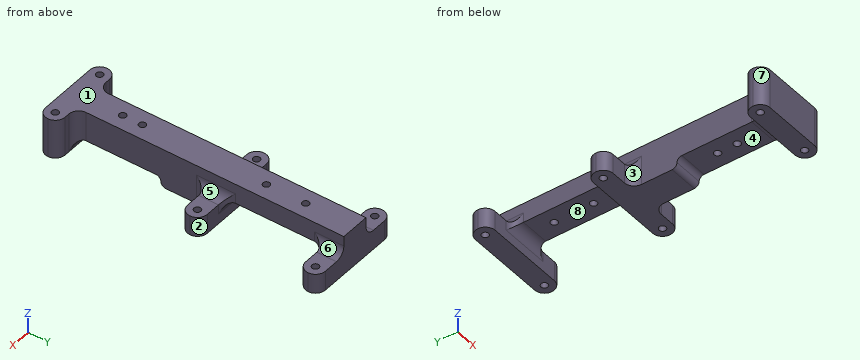
```python
from build123d import *

# Parameters (mm, degrees)
SKETCH1_W                = 50
SKETCH1_H                = 10
BOSS_EXTRUDE1_DEPTH      = 10
BOSS_EXTRUDE1_2_DEPTH    = 10
SKETCH2_W                = 15
SKETCH2_H                = 70
BOSS_EXTRUDE2_DEPTH      = 10
CUT_EXTRUDE1_REACH       = 49.434
SKETCH3_R                = 1.75
CUT_EXTRUDE2_REACH       = 46.159
SKETCH4_R                = 1.75
FILLET2_R                = 5
FILLET4_R                = 5
FILLET5_R                = 5
FILLET6_R                = 5
SKETCH5_W                = 15
SKETCH5_H                = 20
BOSS_EXTRUDE3_DEPTH      = 66
BOSS_EXTRUDE4_DEPTH      = 20
BOSS_EXTRUDE4_DEPTH_BACK = 20
SKETCH6_W                = 20
SKETCH6_H                = 10
CUT_EXTRUDE3_REACH       = 117.525
SKETCH7_R                = 1.75
FILLET7_R                = 5
FILLET9_R                = 5
FILLET10_R               = 5
SKETCH8_R                = 1.75
CUT_EXTRUDE4_DEPTH       = 116.524889093
SKETCH11_W               = 15
SKETCH11_H               = 43
CUT_EXTRUDE5_DEPTH       = 5
FILLET11_R               = 5
FILLET13_R               = 2.5


# Some blends are built 0.0001 mm under size
with BuildPart() as part:
    # Sketch1 → Boss-Extrude1 (new body)
    with BuildSketch(Plane.XY):
        with Locations((0, 30)):
            Rectangle(SKETCH1_W, SKETCH1_H)
    extrude(amount=BOSS_EXTRUDE1_DEPTH)



with BuildPart() as body_2:
    # Sketch1 → Boss-Extrude1 2 (new body)
    with BuildSketch(Plane.XY):
        with Locations((0, -30)):
            Rectangle(SKETCH1_W, SKETCH1_H)
    extrude(amount=BOSS_EXTRUDE1_2_DEPTH)


with BuildPart() as part_1:
    add(part.part)

    add(body_2.part)  # Boss-Extrude2 merges body 2
    # Sketch2 → Boss-Extrude2 (add)
    with BuildSketch(Plane.XY.offset(10)):
        Rectangle(SKETCH2_W, SKETCH2_H)
    extrude(amount=BOSS_EXTRUDE2_DEPTH)

    # Sketch3 → Cut-Extrude1 (cut, up to next)
    with BuildSketch(Plane.XY.offset(20), mode=Mode.PRIVATE) as cut_extrude1_sk1:
        with Locations((0, 10)):
            Circle(SKETCH3_R)
    cut_extrude1_tool1 = extrude(cut_extrude1_sk1.sketch, amount=-CUT_EXTRUDE1_REACH, mode=Mode.PRIVATE) & part_1.part
    # Sketch3 → Cut-Extrude1 (cut, up to next)
    with BuildSketch(Plane.XY.offset(20), mode=Mode.PRIVATE) as cut_extrude1_sk2:
        with Locations((0, -10)):
            Circle(SKETCH3_R)
    cut_extrude1_tool2 = extrude(cut_extrude1_sk2.sketch, amount=-CUT_EXTRUDE1_REACH, mode=Mode.PRIVATE) & part_1.part
    add(cut_extrude1_tool1.solids().sort_by_distance((0, 10, 20))[0], mode=Mode.SUBTRACT)
    add(cut_extrude1_tool2.solids().sort_by_distance((0, -10, 20))[0], mode=Mode.SUBTRACT)

    # Sketch4 → Cut-Extrude2 (cut, up to next)
    with BuildSketch(Plane.XY.offset(10), mode=Mode.PRIVATE) as cut_extrude2_sk1:
        with Locations((-20, 30)):
            Circle(SKETCH4_R)
    cut_extrude2_tool1 = extrude(cut_extrude2_sk1.sketch, amount=-CUT_EXTRUDE2_REACH, mode=Mode.PRIVATE) & part_1.part
    # Sketch4 → Cut-Extrude2 (cut, up to next)
    with BuildSketch(Plane.XY.offset(10), mode=Mode.PRIVATE) as cut_extrude2_sk2:
        with Locations((-20, -30)):
            Circle(SKETCH4_R)
    cut_extrude2_tool2 = extrude(cut_extrude2_sk2.sketch, amount=-CUT_EXTRUDE2_REACH, mode=Mode.PRIVATE) & part_1.part
    # Sketch4 → Cut-Extrude2 (cut, up to next)
    with BuildSketch(Plane.XY.offset(10), mode=Mode.PRIVATE) as cut_extrude2_sk3:
        with Locations((20, 30)):
            Circle(SKETCH4_R)
    cut_extrude2_tool3 = extrude(cut_extrude2_sk3.sketch, amount=-CUT_EXTRUDE2_REACH, mode=Mode.PRIVATE) & part_1.part
    # Sketch4 → Cut-Extrude2 (cut, up to next)
    with BuildSketch(Plane.XY.offset(10), mode=Mode.PRIVATE) as cut_extrude2_sk4:
        with Locations((20, -30)):
            Circle(SKETCH4_R)
    cut_extrude2_tool4 = extrude(cut_extrude2_sk4.sketch, amount=-CUT_EXTRUDE2_REACH, mode=Mode.PRIVATE) & part_1.part
    add(cut_extrude2_tool1.solids().sort_by_distance((-20, 30, 10))[0], mode=Mode.SUBTRACT)
    add(cut_extrude2_tool2.solids().sort_by_distance((-20, -30, 10))[0], mode=Mode.SUBTRACT)
    add(cut_extrude2_tool3.solids().sort_by_distance((20, 30, 10))[0], mode=Mode.SUBTRACT)
    add(cut_extrude2_tool4.solids().sort_by_distance((20, -30, 10))[0], mode=Mode.SUBTRACT)

    # Fillet2
    fillet2_edges = [part_1.edges().sort_by_distance(p)[0] for p in [
        (25, -35, 5),
        (25, -25, 5),
        (25, 35, 5),
        (25, 25, 5),
        (-25, 35, 5),
        (-25, 25, 5),
        (-25, -25, 5),
        (-25, -35, 5),
    ]]
    fillet(fillet2_edges, radius=FILLET2_R - 0.0001)  # a hair under: the kernel refuses the full size

    # Fillet4
    # the kernel refuses this fillet: 5 mm, written as the material it adds along each edge
    with BuildSketch(Plane(origin=(7.5, 25, 10), x_dir=(0, 0, -1), z_dir=(-1, 0, 0))) as fillet4_piece_1:
        with BuildLine():
            CenterArc((FILLET4_R, FILLET4_R), FILLET4_R, 180, 90)
            Line((0, FILLET4_R), (0, 0))
            Line((0, 0), (FILLET4_R, 0))
        make_face()
    extrude(amount=15)
    with BuildSketch(Plane(origin=(-7.5, -25, 10), x_dir=(0, 1, 0), z_dir=(1, 0, 0))) as fillet4_piece_2:
        with BuildLine():
            CenterArc((FILLET4_R, -FILLET4_R), FILLET4_R, 90, 90)
            Line((0, -FILLET4_R), (0, 0))
            Line((0, 0), (FILLET4_R, 0))
        make_face()
    extrude(amount=15)

    # Fillet5
    fillet5_edges = [part_1.edges().sort_by_distance(p)[0] for p in [
        (7.5, -25, 7.5),
        (7.5, 25, 7.5),
    ]]
    fillet(fillet5_edges, radius=FILLET5_R - 0.0001)  # a hair under: the kernel refuses the full size

    # Fillet6
    fillet6_edges = [part_1.edges().sort_by_distance(p)[0] for p in [
        (-7.5, -25, 7.5),
        (-7.5, 25, 7.5),
    ]]
    fillet(fillet6_edges, radius=FILLET6_R - 0.0001)  # a hair under: the kernel refuses the full size

    # Sketch5 → Boss-Extrude3 (add)
    with BuildSketch(Plane.XZ.offset(35)):
        with Locations((0, 10)):
            Rectangle(SKETCH5_W, SKETCH5_H)
    extrude(amount=BOSS_EXTRUDE3_DEPTH)

    # Sketch6 → Boss-Extrude4 (add, two sides: drawn at the far end of the back side and taken through both)
    with BuildSketch(Plane(origin=(0, 0, 0), x_dir=(0, 0, -1), z_dir=(1, 0, 0)).offset(-BOSS_EXTRUDE4_DEPTH_BACK)):
        with Locations((-10, -106)):
            Rectangle(SKETCH6_W, SKETCH6_H)
    extrude(amount=BOSS_EXTRUDE4_DEPTH + BOSS_EXTRUDE4_DEPTH_BACK)

    # Sketch7 → Cut-Extrude3 (cut, up to next)
    with BuildSketch(Plane.XY.offset(20), mode=Mode.PRIVATE) as cut_extrude3_sk1:
        with Locations((-15, -106)):
            Circle(SKETCH7_R)
    cut_extrude3_tool1 = extrude(cut_extrude3_sk1.sketch, amount=-CUT_EXTRUDE3_REACH, mode=Mode.PRIVATE) & part_1.part
    # Sketch7 → Cut-Extrude3 (cut, up to next)
    with BuildSketch(Plane.XY.offset(20), mode=Mode.PRIVATE) as cut_extrude3_sk2:
        with Locations((15, -106)):
            Circle(SKETCH7_R)
    cut_extrude3_tool2 = extrude(cut_extrude3_sk2.sketch, amount=-CUT_EXTRUDE3_REACH, mode=Mode.PRIVATE) & part_1.part
    add(cut_extrude3_tool1.solids().sort_by_distance((-15, -106, 20))[0], mode=Mode.SUBTRACT)
    add(cut_extrude3_tool2.solids().sort_by_distance((15, -106, 20))[0], mode=Mode.SUBTRACT)

    # Fillet7
    fillet7_edges = [part_1.edges().sort_by_distance(p)[0] for p in [
        (20, -111, 10),
        (20, -101, 10),
        (-20, -111, 10),
        (-20, -101, 10),
    ]]
    fillet(fillet7_edges, radius=FILLET7_R - 0.0001)  # a hair under: the kernel refuses the full size

    # Fillet9
    fillet9_edges = [part_1.edges().sort_by_distance(p)[0] for p in [
        (-7.5, -35, 5),
        (7.5, -35, 5),
    ]]
    fillet(fillet9_edges, radius=FILLET9_R)

    # Fillet10
    fillet10_edges = [part_1.edges().sort_by_distance(p)[0] for p in [
        (7.5, -30.00005, 10),
        (7.5, 27.50005, 10),
        (-7.5, -30.00005, 10),
        (-7.5, 27.50005, 10),
    ]]
    fillet(fillet10_edges, radius=FILLET10_R)

    # Sketch8 → Cut-Extrude4 (cut, through all)
    with BuildSketch(Plane.XY.offset(20)):
        with Locations((0, -73)):
            Circle(SKETCH8_R)
        with Locations((0, -83)):
            Circle(SKETCH8_R)
    extrude(amount=-CUT_EXTRUDE4_DEPTH, mode=Mode.SUBTRACT)

    # Sketch11 → Cut-Extrude5 (cut)
    with BuildSketch(Plane(origin=(0, 0, 0), x_dir=(-1, 0, 0), z_dir=(0, 0, -1))):
        with Locations((0, -79.5)):
            Rectangle(SKETCH11_W, SKETCH11_H)
    extrude(amount=-CUT_EXTRUDE5_DEPTH, mode=Mode.SUBTRACT)

    # Fillet11
    fillet11_edges = [part_1.edges().sort_by_distance(p)[0] for p in [
        (-7.5, -101, 12.5),
        (7.5, -101, 12.5),
        (0, -101, 5),
    ]]
    fillet(fillet11_edges, radius=FILLET11_R - 0.0001)  # a hair under: the kernel refuses the full size

    # Fillet13
    fillet13_edges = [part_1.edges().sort_by_distance(p)[0] for p in [
        (0, -58, 5),
    ]]
    fillet(fillet13_edges, radius=FILLET13_R)
    fillet13_2_edges = [part_1.edges().sort_by_distance(p)[0] for p in [
        (0, -58, 0),
    ]]
    fillet(fillet13_2_edges, radius=FILLET13_R - 0.0001)  # a hair under: the kernel refuses the full size


solid = part_1.part
```
Here's how the part is built. I have some questions about the finished solid (model axes, mm). Face numbers are marked on the shaded views. A direction names the side the tool comes from. Coordinates: 2 decimals unless noted, no trailing zeros. Order: outer loops, then holes, each group sorted by start corner. A loop starts at its lowest first (then second) coordinate and runs counter-clockwise, first axis right, second up. Notation, with made-up numbers: (22, -35) - (78, -35) arc R17 ccw to (78, -23) - close; hole circle Ø3 at (19, -7.5). An arc over 180 degrees is marked (long way). One line per question, with ' | ' between items.
(1) If we mould it in two halves opening along Y, with no side actions, what happens to the marked faces 6, 7 and 8? For each: pulls with the +Y half, pulls with the -Y half, needs draft (parallel to the pull), parting line crosses it, or undercut.
Report:
face 6: needs draft | face 7: pulls with the -Y half | face 8: undercut
(2) Suppose I cut it at C-C on y = -41.5. List the corners of the cut face in (x, z) for me, and give its area (3 significant figures).
Report:
outline: (-7.5, 0) - (7.5, 0) - (7.5, 20) - (-7.5, 20) - close | area: 300 mm2
(3) Will these pins go through, and if not, where does the flat tip stop? pin 1 (1 mm diameter, centred on y = 17, z = 14.5, fed in from +X); pin 2 (12 mm diameter, centred on x = 13, y = -13.5, fed in from -Z); pin 3 (4 mm diameter, centred on x = 20, y = -30, fed in from +Z).
Report:
pin 1: stops at x = 7.5 | pin 2: stops at z = 10 | pin 3: stops at z = 10
(4) Suppose I cut it at A-A on x = 0. State how many separate pieces and enclosed holes the cut face has, and give its area (3 significant figures).
Report:
separate pieces: 5 | enclosed holes: 0 | area: 2,050 mm2
(5) For the marked faces 1, 2, 3, 4 and 5, which set-ups out of +Z, -Z, +X, -X, +Y, -Y let a thin tool reach every point of the face, with its end or its side?
Report:
face 1: +Z, +X, -X, +Y, -Y | face 2: +Z, -Z, +X | face 3: +Z, -Z, -X | face 4: -Z, +X, -X | face 5: +Z, +X, +Y
(6) Suppose I cut it at D-D on y = 1.5. List the corners of the cut face in (x, z) for me, and give its area (3 significant figures).
Report:
outline: (-7.5, 10) - (7.5, 10) - (7.5, 20) - (-7.5, 20) - close | area: 150 mm2
(7) If I drill on L1, parallel to X at y = -106, z = 8.5; L2, parallel to Y at x = 0, z = 11; L3, parallel to Y at x = -15, z = 8, over which ranges is the centre line in solid material (lowest first)?
Report:
L1: x = -20 to -16.75, -13.25 to 13.25, 16.75 to 20 | L2: y = -111 to -84.75, -81.25 to -74.75, -71.25 to -11.75, -8.25 to 8.25, 11.75 to 35 | L3: y = -111 to -107.75, -104.25 to -101, -35 to -25, 25 to 35
